Part model, mm, in its own coordinate system. A direction names the side the tool comes from. Give positions to 0.01 mm unless a question says otherwise; leave off trailing zeros. Write each loop counter-clockwise with the first axis right and the second up, starting at its lowest first coordinate (ties: lowest second). Pieces come first, ordered by that corner, then holes. Notation, with made-up numbers: M 33.25,74 L 67.25,74 A21 cw 67.25,105 Z; hole C 31,74 d6. An arc over 180 degrees is marked long. Use CSV: the item, a comma, the result in double quotes. Start each with the question number.
Item 1: Cut at B-B (z = 33). List the corners of the cut face in (x, y) (3 decimals).
Item 2: Cut at A-A (x = 0). List the corners of the cut face in (y, z), then the cut area to 3 significant figures.
Item 3: Drill centre lines: line 1 (Y direction, x = 0, z = 1); line 2 (X direction, y = -51, z = 20); line 3 (X direction, y = 63, z = 3). Where is each one in solid material? Low to high. Write a range as [from, to].
Item 4: Which spindle directions (+Z, -Z, +X, -X, +Y, -Y) get a long thin tool onto all of the face, cutting with end or side? Do faces 1 (the flat face through (-43, 24, 55)), 2 (the cylindrical face through (45.03, 77.92, 30.42)). Say none if no direction does.
Item 5: Mould opens along Y. For faces 3 (the cylindrical face through (-45.117, 78.036, 30.42)), 4 (the flat face through (45, 25, 60)), 5 (the flat face through (0, -72.607, 29)) say: released by +Y, released by -Y, zero draft, split by the parting line, or undercut.
Item 6: Cut at C-C (x = -15). List the corners of the cut face in (y, z).
Item 7: Pin check, flat tips, straight feed: pin 1 (2 mm diameter, centred on y = -47, z = 43.5, fed in from -X); pin 2 (12 mm diameter, centred on y = -2, z = 25, fed in from +X); pin 3 (15 mm diameter, centred on x = 0, y = -50.63, fed in from -Z); pin 4 (3 mm diameter, centred on y = 24, z = 22.5, fed in from -X). Stop position of each tip, or through.
Item 8: Cut at D-D (y = -46). List the corners of the cut face in (x, z).
from build123d import *

# Parameters (mm, degrees)
F1_DEPTH = 60
F2_DEPTH = 55
F0_R     = 27.667587
F0_R_2   = 24.667588
F3_DEPTH = 4
F0_R_3   = 6.567471
F4_DEPTH = 2.9
F5_R     = 7.261182


with BuildPart() as f1:
    # F0 (on Top) → F1 (new body)
    with BuildSketch(Plane.XY):
        Polygon((47.330219, -78.107089), (47.093301, 80.102593), (-47.29298, 80.102593), (-47.530543, -78.107089), align=None)
        Polygon((-44.526036, -75.10709), (-44.297483, 77.102594), (44.097792, 77.102594), (44.325725, -75.10709), align=None, mode=Mode.SUBTRACT)
    extrude(amount=F1_DEPTH)

    # F0 (on Top) → F2 (join)
    with BuildSketch(Plane.XY):
        Polygon((44.097792, 77.102594), (-44.297483, 77.102594), (-44.526036, -75.10709), (44.325725, -75.10709), align=None)
        Polygon((-42.02228, -72.60709), (-41.801234, 74.602594), (41.601533, 74.602594), (41.821978, -72.60709), align=None, mode=Mode.SUBTRACT)
    extrude(amount=F2_DEPTH)



with BuildPart() as f3:
    # F0 (on Top) → F3 (new body)
    with BuildSketch(Plane.XY):
        with Locations((0, 44.681013)):
            Circle(F0_R)
        with Locations((0, 44.681013)):
            Circle(F0_R_2, mode=Mode.SUBTRACT)
    extrude(amount=F3_DEPTH)


with BuildPart() as f1_1:
    add(f1.part)

    add(f3.part)  # F4 merges F3
    # F0 (on Top) → F4 (join)
    with BuildSketch(Plane.XY):
        Polygon((41.601533, 74.602594), (-41.801234, 74.602594), (-42.02228, -72.60709), (41.821978, -72.60709), align=None)
        with Locations((0, -50.630033)):
            Circle(F0_R_3, mode=Mode.SUBTRACT)
        with Locations((0, 44.681013)):
            Circle(F0_R, mode=Mode.SUBTRACT)
    extrude(amount=F4_DEPTH)

    # F5
    f5_edges = [f1_1.edges().sort_by_distance(p)[0] for p in [
        (47.330219, -78.107089, 30),
        (-47.530543, -78.107089, 30),
        (-47.29298, 80.102593, 30),
        (47.093301, 80.102593, 30),
    ]]
    fillet(f5_edges, radius=F5_R)


solid = f1_1.part
Worked answers:
1,outline,"M -47.52,-70.835 A7.261 ccw -40.258,-78.107 L 40.058,-78.107 A7.261 ccw 47.319,-70.835 L 47.104,72.852 A7.261 ccw 39.843,80.103 L -40.043,80.103 A7.261 ccw -47.304,72.852 Z; hole M -42.022,-72.607 L 41.822,-72.607 L 41.602,74.603 L -41.801,74.603 Z"
2,outline,"M -78.11,0 L -57.2,0 L -57.2,2.9 L -72.61,2.9 L -72.61,55 L -75.11,55 L -75.11,60 L -78.11,60 Z; M -44.06,0 L 20.01,0 L 20.01,4 L 17.01,4 L 17.01,2.9 L -44.06,2.9 Z; M 69.35,0 L 80.1,0 L 80.1,60 L 77.1,60 L 77.1,55 L 74.6,55 L 74.6,2.9 L 72.35,2.9 L 72.35,4 L 69.35,4 Z"
2,area,"887 mm^2"
3,line 1,"y = [-78.11, -57.2], [-44.06, 20.01], [69.35, 80.1]"
3,line 2,"x = [-47.49, -41.99], [41.79, 47.29]"
3,line 3,"x = [-47.32, -41.82], [-20.73, -16.52], [16.52, 20.73], [41.62, 47.12]"
4,face 1,"+Z"
4,face 2,"+Z, -Z, +X, +Y"
5,face 3,"released by +Y"
5,face 4,"zero draft"
5,face 5,"undercut"
6,outline,"M -78.11,0 L 25.1,0 L 25.1,4 L 21.43,4 L 21.43,2.9 L -72.61,2.9 L -72.61,55 L -75.11,55 L -75.11,60 L -78.11,60 Z; M 64.26,0 L 80.1,0 L 80.1,60 L 77.1,60 L 77.1,55 L 74.6,55 L 74.6,2.9 L 67.93,2.9 L 67.93,4 L 64.26,4 Z"
7,pin 1,"stops at x = -47.49"
7,pin 2,"stops at x = 47.23"
7,pin 3,"stops at z = 0"
7,pin 4,"stops at x = -47.38"
8,outline,"M -47.48,0 L -4.66,0 L -4.66,2.9 L -41.98,2.9 L -41.98,55 L -44.48,55 L -44.48,60 L -47.48,60 Z; M 4.66,0 L 47.28,0 L 47.28,60 L 44.28,60 L 44.28,55 L 41.78,55 L 41.78,2.9 L 4.66,2.9 Z"
